from build123d import *

# Parameters (mm, degrees)
SKETCH1_R           = 78.359
SKETCH1_R_2         = 76.2
BOSS_EXTRUDE1_DEPTH = 609.6
CUT_EXTRUDE1_START  = -381
CUT_EXTRUDE1_DEPTH  = 381
CIRPATTERN1_COUNT   = 3


with BuildPart() as part:
    # Sketch1 → Boss-Extrude1 (new body)
    with BuildSketch(Plane(origin=(0, 0, 0), x_dir=(0, 0, -1), z_dir=(1, 0, 0))):
        with Locations(Location((0, 0, 0), (0, 0, 180))):
            Circle(SKETCH1_R)
        with Locations(Location((0, 0, 0), (0, 0, 180))):
            Circle(SKETCH1_R_2, mode=Mode.SUBTRACT)
    extrude(amount=BOSS_EXTRUDE1_DEPTH)

    # Sketch3 → Cut-Extrude1 (cut)
    with BuildSketch(Plane(origin=(577.85, 0, 0), x_dir=(0, 0, -1), z_dir=(1, 0, 0)).offset(CUT_EXTRUDE1_START)):
        with BuildLine():
            Line((-3.175, 78.294650239), (-3.175, 76.133825433))
            ThreePointArc((-3.175, 76.133825433), (0, 76.2), (3.175, 76.133825433))
            Line((3.175, 76.133825433), (3.175, 78.294650239))
            ThreePointArc((3.175, 78.294650239), (0, 78.359), (-3.175, 78.294650239))
        make_face()
    cut_extrude1 = extrude(amount=CUT_EXTRUDE1_DEPTH, mode=Mode.SUBTRACT)

    # CirPattern1: Cut-Extrude1 ×3 about axis
    cirpattern1_axis = Axis((0, 0, 0), (1, 0, 0))
    for i in range(1, CIRPATTERN1_COUNT):
        add(cut_extrude1.rotate(cirpattern1_axis, i * 360 / CIRPATTERN1_COUNT), mode=Mode.SUBTRACT)


solid = part.part
Input: part model. Units: mm. Frame: model coordinates. Give positions to 0.01 mm unless a question says otherwise; leave off trailing zeros. Write each loop counter-clockwise with the first axis right and the second up, starting at its lowest first coordinate (ties: lowest second). Pieces come first, ordered by that corner, then holes.
Q1. Section C-C, the plane z = -21. Output: boundary loops of the cut face in (x, y).
Q2. Material intervals for probe 1 along Y at (x, z) = (144, 0); probe 2 along Z at (x, y) = (580.5, 3.5); probe 3 along Y at (x, z) = (419.5, 0), sorted ascending.
Q3. Section A-A, the plane x = 250.5. Output: boundary loops of the cut face in (y, z) (3 decimals).
Q4. Section B-B, the plane y = -19. Output: boundary loops of the cut face in (x, z), plus the area to 3 significant figures.
Q5. Pull-direction query (Y, two-part tool) for faces 1 (the face through (609.6, 75, 17)), 2 (the face through (300.53, -23.54, 74.74)), 3 (the face through (300.533, 74.388, -16.519)); classes: pulls with the +Y half, pulls with the -Y half, needs draft (parallel to the pull), parting line crosses it, or undercut.
Q6. First-contact query: P1, Ø1.5, axis at x = 504, z = -32, coming from the +Y side; P2, Ø5, axis at x = 205, z = 43, coming from the -Y side; P3, Ø4, axis at x = 374, y = -6, coming from the +Z side. Flat tips, straight axial feed; report the tip coordinate or a pass-through.
Filled in:
1. outline: (0, -75.49) - (609.6, -75.49) - (609.6, -73.25) - (0, -73.25) - close; (0, 73.25) - (609.6, 73.25) - (609.6, 75.49) - (0, 75.49) - close
2. probe 1: y = -78.36 to -76.2, 76.2 to 78.36
2. probe 2: z = -78.28 to -76.12, 76.12 to 78.28
2. probe 3: y = -78.36 to -76.2
3. outline: (-41.897, -66.218) - (-40.817, -64.346) arc R76.2 cw to (-40.817, 64.346) - (-41.897, 66.218) arc R78.359 ccw to start; (-36.398, -69.393) arc R78.359 ccw to (78.295, -3.175) - (76.134, -3.175) arc R76.2 cw to (-35.317, -67.521) - close; (-36.398, 69.393) - (-35.317, 67.521) arc R76.2 cw to (76.134, 3.175) - (78.295, 3.175) arc R78.359 ccw to start
4. outline: (0, -76.02) - (609.6, -76.02) - (609.6, -73.79) - (0, -73.79) - close; (0, 73.79) - (609.6, 73.79) - (609.6, 76.02) - (0, 76.02) - close
4. area: 2,720 mm2
5. face 1: needs draft
5. face 2: parting line crosses it
5. face 3: undercut
6. P1: stops at y = 71.86
6. P2: stops at y = -67.08
6. P3: stops at z = 78.26
